Read the model definition and answer for the solid it produces. Units are mm, in the model's axes. A direction names the side the tool comes from. Give positions to 0.01 mm unless a question says otherwise; leave off trailing zeros. Order: outer loops, then holes, each group sorted by start corner. A loop starts at its lowest first (then second) coordinate and runs counter-clockwise, first axis right, second up. Notation, with made-up numbers: M -35,87 L 9,87 A10 cw 9,95 Z; hole C 69,-2.5 d10. An arc over 180 degrees is marked long. One line per item, written item: value.
from build123d import *

# Parameters (mm, degrees)
SKETCH2_W          = 10.16
SKETCH2_H          = 12.7
SKETCH3_W          = 10.16
SKETCH3_H          = 12.7
CUT_EXTRUDE1_DEPTH = 5.08
SKETCH5_R          = 5.092900553
CUT_EXTRUDE2_DEPTH = 127


with BuildPart() as part:
    # Sweep2: sweep along a path in Sketch1
    with BuildLine(Plane.XY) as sweep2_path:
        Line((0, 0), (-16.795144912, 95.25))
        ThreePointArc((-16.795144912, 95.25), (-13.064303558, 109.17368949), (0, 115.265674288))
        Line((0, 115.265674288), (68.58, 115.265674288))
        ThreePointArc((68.58, 115.265674288), (81.644303558, 109.17368949), (85.375144912, 95.25))
        Line((85.375144912, 95.25), (68.58, 0))
    # Sketch2 → Sweep2 (sweep)
    with BuildSketch(Plane(origin=(0, 0, 0), x_dir=(1, 0, 0), z_dir=(0, 1, 0))):
        with Locations((-5.08, 0)):
            Rectangle(SKETCH2_W, SKETCH2_H)
    sweep(path=sweep2_path.line)

    # Sketch3 → Cut-Extrude1 (cut)
    with BuildSketch(Plane(origin=(0, 0, 0), x_dir=(1, 0, 0), z_dir=(0, 1, 0))):
        with Locations((73.66, 0)):
            Rectangle(SKETCH3_W, SKETCH3_H)
    extrude(amount=-CUT_EXTRUDE1_DEPTH, mode=Mode.SUBTRACT)

    # Sketch5 → Cut-Extrude2 (cut, symmetric)
    with BuildSketch(Plane(origin=(0, 0, 0), x_dir=(0, 0, -1), z_dir=(1, 0, 0))):
        with Locations(Location((0, 12.7, 0), (0, 0, 270))):
            Circle(SKETCH5_R)
    extrude(amount=CUT_EXTRUDE2_DEPTH, both=True, mode=Mode.SUBTRACT)


solid = part.part
1) Determine the mould class of faces 1 (the face through (74, 0, 0)), 2 (the face through (76.026, 7.842, -1.53)), 3 (the face through (-7.277, 7.842, -1.53)), 4 (the face through (35, 119, -6.35)) for opening direction Z: +Z half, -Z half, draft (parallel to the pull), parting line (faces both ways), or undercut.
Reported:
face 1: draft
face 2: undercut
face 3: undercut
face 4: -Z half
2) Find section A-A, the plane z = 1.75. Write down the section's boundary in (x, y).
Reported:
outline: M -26.96,95.25 L -13.24,17.48 L -3.08,17.48 L -16.8,95.25 A17.05 cw 0,115.27 L 68.58,115.27 A17.05 cw 85.38,95.25 L 71.66,17.48 L 81.82,17.48 L 94.92,91.78 A27.12 ccw 70.34,125.27 L 1.76,125.27 A27.12 ccw Z; M -11.56,7.92 L -10.16,0 L 0,0 L -1.4,7.92 Z; M 68.58,0 L 78.74,0 L 80.14,7.92 L 69.98,7.92 Z
3) Consider probe 1 along Z at (x, y) = (72.75, 12.7); probe 2 along Y at (x, z) = (17.5, 3.25). Determine where each line is inside the solid, lowest interval first.
Reported:
probe 1: z = -6.35 to -5.09, 5.09 to 6.35
probe 2: y = 115.27 to 125.27
4) Find section B-B, the plane y = 49.5. Write down the section's boundary in (x, z).
Reported:
outline: M -18.89,-6.35 L -8.73,-6.35 L -8.73,6.35 L -18.89,6.35 Z; M 77.31,-6.35 L 87.47,-6.35 L 87.47,6.35 L 77.31,6.35 Z
5) Find section D-D, the plane x = 50.5. Write down the section's boundary in (y, z), plus the area to 3 significant figures.
Reported:
outline: M 115.27,-6.35 L 125.27,-6.35 L 125.27,6.35 L 115.27,6.35 Z
area: 127 mm^2
6) Each of these flat-tipped pins is pushed along its axis until it touches: pin 1 Ø2 at (x, z) = (-5, 2.5) entering from +Y; pin 2 Ø5 at (x, z) = (15.5, -4.5) entering from +Y; pin 3 Ø1 at (y, z) = (70, 5) entering from +X. Where does it stop, or does it pass through?
Reported:
pin 1: stops at y = 125.03
pin 2: stops at y = 125.27
pin 3: stops at x = 91.17
7) Which of the six approach directions +Z, -Z, +X, -X, +Y, -Y give full straight-line access (tool end or side, diameter ignored) to faces 5 (the face through (-5, 0, 0)), 6 (the face through (35, 115.266, 0)), 7 (the face through (-8.515, 48.292, 0.089))?
Reported:
face 5: +Z, -Z, +X, -X, -Y
face 6: +Z, -Z, -Y
face 7: +Z, -Z
8) Find section C-C, the plane y = 9.5. Write down the section's boundary in (x, z), plus the area to 3 significant figures.
Reported:
outline: M -11.84,-6.35 L -1.68,-6.35 L -1.68,-3.96 L -11.84,-3.96 Z; M -11.84,3.96 L -1.68,3.96 L -1.68,6.35 L -11.84,6.35 Z; M 70.26,-6.35 L 80.42,-6.35 L 80.42,-3.96 L 70.26,-3.96 Z; M 70.26,3.96 L 80.42,3.96 L 80.42,6.35 L 70.26,6.35 Z
area: 97.0 mm^2
